```python
from build123d import *

# Parameters (mm, degrees)
SKETCH_1_W          = 150
SKETCH_1_H          = 80
EXTRUDE_1_DEPTH     = 25
CUT_EXTRUDE_1_DEPTH = 15
MOVE_BODY_1_ANGLE   = 90


with BuildPart() as part:
    # 草图1 → 凸台-拉伸1 (new body)
    with BuildSketch(Plane(origin=(0, 0, 0), x_dir=(1, 0, 0), z_dir=(0, 1, 0))):
        Rectangle(SKETCH_1_W, SKETCH_1_H)
    extrude(amount=EXTRUDE_1_DEPTH)

    # 草图2 → 切除-拉伸1 (cut)
    with BuildSketch(Plane(origin=(0, 25, 0), x_dir=(1, 0, 0), z_dir=(0, 1, 0))):
        with BuildLine():
            Line((-32.5, 20), (32.5, 20))
            ThreePointArc((32.5, 20), (52.5, 0), (32.5, -20))
            Line((32.5, -20), (-32.5, -20))
            ThreePointArc((-32.5, -20), (-52.5, 0), (-32.5, 20))
        make_face()
    extrude(amount=-CUT_EXTRUDE_1_DEPTH, mode=Mode.SUBTRACT)


with BuildPart() as part_1:
    # Move Body 1: moved
    add(part.part.rotate(Axis((0, 12.5, 0), (1, 0, 0)), MOVE_BODY_1_ANGLE))


solid = part_1.part
```
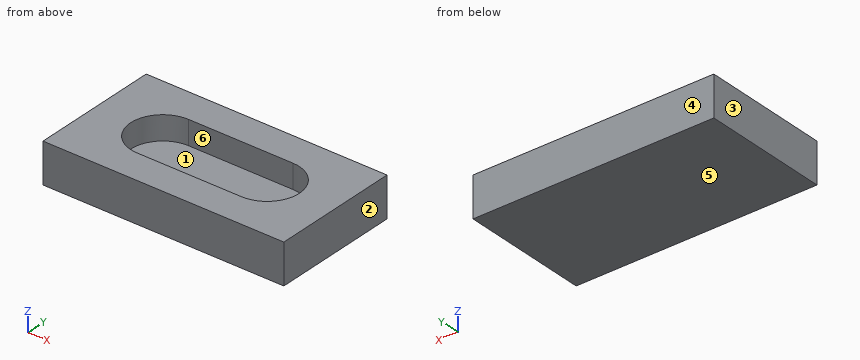
Design review of the part built by this model. Coordinates are the model's own, in mm. Face numbers are marked on the shaded views. A direction names the side the tool comes from. Give positions to 0.01 mm unless a question says otherwise; leave off trailing zeros. Loops run counter-clockwise (first coordinate to the right, second up) from the corner with the lowest first, then second, coordinate; pieces in that order, holes last. Notation, with made-up numbers: M -25,86.5 L 27,86.5 A8 cw 27,98.5 Z; hole C -39.75,3 d8. An arc over 180 degrees is marked long. Return JSON: item names as keys, results as strings. Group by question number.
Item 1: For probe 1 along Y at (x, z) = (-12, 9); probe 2 along X at (y, z) = (11.5, -0.75); probe 3 along Z at (x, y) = (-29, 27), list the stretches that pass through material, from the lowest coordinate up.
Item 2: We need section B-B (y = 12.5). Give the boundary of the cut face in (x, z), and give its area (4 significant figures).
Item 3: We need section C-C (x = 24.5). Give the boundary of the cut face in (y, z), and give its area (3 significant figures).
Item 4: Insertion check: pin 1 Ø1.5 at (x, y) = (-6.5, 17.5) entering from +Z. The pin has a flat end and moves straight along its axis. Give the tip position at first contact, or say it passes through.
Item 5: We need section A-A (z = 0.75). Give the boundary of the cut face in (x, y), and give its area (3 significant figures).
Item 6: Tool access review of the marked faces 5 and 6: name each direction out of +Z, -Z, +X, -X, +Y, -Y from which nothing blocks a thin tool from reaching the whole face with its end or side.
Item 7: Mouldability with a two-part tool opening along X and no side actions: class the marked faces 1, 2, 3 and 4 as released by +X, released by -X, zero draft, split by the parting line, or undercut.
Output:
{
 "1": {"probe 1": "y = -27.5 to -7.5, 32.5 to 52.5", "probe 2": "x = -75 to -52.47, 52.47 to 75", "probe 3": "z = -12.5 to -2.5"},
 "2": {"outline": "M -75,-12.5 L 75,-12.5 L 75,12.5 L 52.5,12.5 L 52.5,-2.5 L -52.5,-2.5 L -52.5,12.5 L -75,12.5 Z", "area": "2,175 mm^2"},
 "3": {"outline": "M -27.5,-12.5 L 52.5,-12.5 L 52.5,12.5 L 32.5,12.5 L 32.5,-2.5 L -7.5,-2.5 L -7.5,12.5 L -27.5,12.5 Z", "area": "1,400 mm^2"},
 "4": {"pin 1": "stops at z = -2.5"},
 "5": {"outline": "M -75,-27.5 L 75,-27.5 L 75,52.5 L -75,52.5 Z; hole M -32.5,-7.5 L 32.5,-7.5 A20 ccw 32.5,32.5 L -32.5,32.5 A20 ccw Z", "area": "8,140 mm^2"},
 "6": {"face 5": "-Z, +X, -X, +Y, -Y", "face 6": "+Z"},
 "7": {"face 1": "undercut", "face 2": "released by +X", "face 3": "released by -X", "face 4": "zero draft"}
}
